Read the model definition and answer for the solid it produces. Units are mm, in the model's axes. A direction names the side the tool comes from. Coordinates: 2 decimals unless noted, no trailing zeros. Loops run counter-clockwise (first coordinate to the right, second up) from the corner with the lowest first, then second, coordinate; pieces in that order, holes last. Notation, with made-up numbers: (-32, 56) -> (-5, 56) arc R32 cw to (-5, 95) -> close; hole circle Ø2 at (21, 27). An arc over 180 degrees is marked (long way). Answer as a JSON object with one key per item and string values. Group by question number.
Q1. Straight lines are drawn through the part: line 1 along X through (y, z) = (-128.5, 0.8); line 2 along X through (y, z) = (-72, 3); line 3 along Y through (x, z) = (19, 1.45). For each, find the intervals that lie inside material, in ascending order. Write a range as [from, to].
Q2. Determine the mould class of faces 3 (the cylindrical face through (0.901, 24.984, 1.972)), 4 (the cylindrical face through (-20.6, -1.2, 2)), 5 (the flat face through (13.435, -67, 2)) for opening direction Y: released by +Y, released by -Y, zero draft, split by the parting line, or undercut.
Q3. The part is cut by section B-B on y = -7. Write down the section's boundary in (x, z).
Q4. For faces 1 (the cylindrical face through (-12.36, -11.75, 1.97)), 2 (the flat face through (-13.435, -65, 2)), determine the directions among +Z, -Z, +X, -X, +Y, -Y from which every point of the face is accessible in a straight line to the end or side of a thin tool.
Q5. The part is cut by section C-C on y = -201.5. Write down the section's boundary in (x, z).
Q6. The part is cut by section A-A on z = 2.1. State how many separate pieces and enclosed holes the cut face has, and give its area (3 significant figures).
Q7. Each of these flat-tipped pins is pushed along its axis until it touches: P1, Ø1, axis at y = -175, z = 2, coming from the +X side; P2, Ø1, axis at x = 7.5, z = 2, coming from the +Y side; P3, Ø2, axis at x = -18.5, z = 2.5, coming from the -Y side; P4, Ø6.5, axis at x = -13.44, y = -13.44, coming from the +Z side. Where does it stop, or does it pass through?
from build123d import *

# Parameters (mm, degrees)
SKETCH_1_R      = 14
SKETCH_1_R_2    = 2
EXTRUDE_1_DEPTH = 4


with BuildPart() as part:
    # 草图1 → 凸台-拉伸1 (new body)
    with BuildSketch(Plane.XY):
        with BuildLine():
            Line((-13.435028843, -21.083168642), (-13.435028843, -111.083168642))
            Line((-13.435028843, -111.083168642), (0, -230))
            Line((0, -230), (13.435028843, -111.083168642))
            Line((13.435028843, -111.083168642), (13.435028843, -21.083168642))
            ThreePointArc((13.435028843, -21.083168642), (0, 25), (-13.435028843, -21.083168642))
        make_face()
        Circle(SKETCH_1_R, mode=Mode.SUBTRACT)
        with Locations((0, 19)):
            Circle(SKETCH_1_R_2, mode=Mode.SUBTRACT)
        with Locations((13.435028843, 13.435028843)):
            Circle(SKETCH_1_R_2, mode=Mode.SUBTRACT)
        with Locations((19, 0)):
            Circle(SKETCH_1_R_2, mode=Mode.SUBTRACT)
        with Locations((13.435028843, -13.435028843)):
            Circle(SKETCH_1_R_2, mode=Mode.SUBTRACT)
        with Locations((0, -19)):
            Circle(SKETCH_1_R_2, mode=Mode.SUBTRACT)
        with Locations((-13.435028843, -13.435028843)):
            Circle(SKETCH_1_R_2, mode=Mode.SUBTRACT)
        with Locations((-19, 0)):
            Circle(SKETCH_1_R_2, mode=Mode.SUBTRACT)
        with Locations((-13.435028843, 13.435028843)):
            Circle(SKETCH_1_R_2, mode=Mode.SUBTRACT)
    extrude(amount=EXTRUDE_1_DEPTH)


solid = part.part
Final values:
{
 "1": {"line 1": "x = [-11.47, 11.47]", "line 2": "x = [-13.44, 13.44]", "line 3": "y = [-16.25, -2], [2, 16.25]"},
 "2": {"face 3": "split by the parting line", "face 4": "undercut", "face 5": "zero draft"},
 "3": {"outline": "(-24, 0) -> (-12.12, 0) -> (-12.12, 4) -> (-24, 4) -> close; (12.12, 0) -> (24, 0) -> (24, 4) -> (12.12, 4) -> close"},
 "4": {"face 1": "+Z, -Z", "face 2": "+Z, -Z, -X, -Y"},
 "5": {"outline": "(-3.22, 0) -> (3.22, 0) -> (3.22, 4) -> (-3.22, 4) -> close"},
 "6": {"separate pieces": "1", "enclosed holes": "9", "area": "5,190 mm2"},
 "7": {"P1": "stops at x = 6.27", "P2": "stops at y = 24", "P3": "stops at y = -17.85", "P4": "stops at z = 4"}
}
